```python
from build123d import *

# Parameters (mm, degrees)
ESQUISSE1_W                                       = 60
ESQUISSE1_H                                       = 22.8
BOSS_EXTRU_1_DEPTH                                = 1.5
ESQUISSE2_W                                       = 60
ESQUISSE2_H                                       = 5
BOSS_EXTRU_2_DEPTH                                = 10
ESQUISSE7_W                                       = 60
ESQUISSE7_H                                       = 22.4
BOSS_EXTRU_3_DEPTH                                = 5
DIAM_TRE_DU_PER_AGE_3_0_3_2_AT_2_COUNT            = 2
DIAM_TRE_DU_PER_AGE_3_0_3_2_AT_2_PITCH            = 10
DIAM_TRE_DU_PER_AGE_3_0_3_2_AT_3_COUNT            = 2
DIAM_TRE_DU_PER_AGE_3_0_3_2_AT_3_PITCH            = 20
DIAM_TRE_DU_PER_AGE_3_0_3_2_AT_4_COUNT            = 2
DIAM_TRE_DU_PER_AGE_3_0_3_2_AT_4_PITCH            = 30
DIAM_TRE_DU_PER_AGE_3_0_3_2_AT_5_COUNT            = 2
DIAM_TRE_DU_PER_AGE_3_0_3_2_AT_5_PITCH            = 40
R_P_TITION_LIN_AIRE2_COUNT                        = 2
R_P_TITION_LIN_AIRE2_PITCH                        = 10
CHAMBRAGE_POUR_VIS_SIX_PANS_CREUX_M31_D           = 3.4
CHAMBRAGE_POUR_VIS_SIX_PANS_CREUX_M31_DEPTH       = 13
CHAMBRAGE_POUR_VIS_SIX_PANS_CREUX_M31_CBORE_D     = 6.5
CHAMBRAGE_POUR_VIS_SIX_PANS_CREUX_M31_CBORE_DEPTH = 1
CHAMBRAGE_POUR_VIS_SIX_PANS_CREUX_M31_TIP         = 1.021463052
R_P_TITION_LIN_AIRE1_COUNT                        = 3
R_P_TITION_LIN_AIRE1_PITCH                        = 10
ESQUISSE10_W                                      = 40
ESQUISSE10_H                                      = 32.8
BOSS_EXTRU_4_DEPTH                                = 2
ESQUISSE11_W                                      = 20
ESQUISSE11_H                                      = 10
ENL_V_MAT_EXTRU_1_DEPTH                           = 17.4
ENL_V_MAT_EXTRU_1_DEPTH_BACK                      = 17.4
ESQUISSE12_R                                      = 4
ESQUISSE12_W                                      = 11.5
ESQUISSE12_H                                      = 8
ENL_V_MAT_EXTRU_2_DEPTH                           = 23.9
ENL_V_MAT_EXTRU_2_DEPTH_BACK                      = 12.5
BOSS_EXTRU_5_DEPTH                                = 4
ESQUISSE14_W                                      = 2
ESQUISSE14_H                                      = 8
ENL_V_MAT_EXTRU_3_DEPTH                           = 1
ENL_V_MAT_EXTRU_3_DEPTH_BACK                      = 65
CONG_2_R                                          = 2
ESQUISSE15_W                                      = 14.8
ESQUISSE15_H                                      = 1.5
ENL_V_MAT_EXTRU_4_DEPTH                           = 5
ENL_V_MAT_EXTRU_4_DEPTH_BACK                      = 25
CONG_3_R                                          = 0.5


with BuildPart() as part:
    # Esquisse1 → Boss.-Extru.1 (new body, symmetric)
    with BuildSketch(Plane(origin=(0, 0, 0), x_dir=(1, 0, 0), z_dir=(0, 1, 0))):
        Rectangle(ESQUISSE1_W, ESQUISSE1_H)
    extrude(amount=BOSS_EXTRU_1_DEPTH, both=True)

    # Esquisse2 → Boss.-Extru.2 (add)
    with BuildSketch(Plane.XZ.offset(1.5)):
        Rectangle(ESQUISSE2_W, ESQUISSE2_H)
    extrude(amount=BOSS_EXTRU_2_DEPTH)

    # Esquisse7 → Boss.-Extru.3 (add)
    with BuildSketch(Plane(origin=(0, 0, -11.4), x_dir=(-1, 0, 0), z_dir=(0, 0, -1))):
        with Locations((0, 9.7)):
            Rectangle(ESQUISSE7_W, ESQUISSE7_H)
    boss_extru_3 = extrude(amount=BOSS_EXTRU_3_DEPTH)

    # Esquisse9 → Diamètre du perçage Ø3.0 (3)2 (revolve, cut)
    with BuildSketch(Plane(origin=(20, 4.5, -16.4), x_dir=(0, 1, 0), z_dir=(1, 0, 0))):
        Polygon((0, 0), (0, 13.901290929), (1.5, 13), (1.5, 0), align=None)
    diam_tre_du_per_age_3_0_3_2 = revolve(axis=Axis((20, 4.5, -22.75), (0, 0, 1)), mode=Mode.SUBTRACT)

    # Diamètre du perçage Ø3.0 (3)2 at 2: Diamètre du perçage Ø3.0 (3)2 ×2
    with Locations(*[(-i * DIAM_TRE_DU_PER_AGE_3_0_3_2_AT_2_PITCH, 0, 0) for i in range(1, DIAM_TRE_DU_PER_AGE_3_0_3_2_AT_2_COUNT)]):
        add(diam_tre_du_per_age_3_0_3_2, mode=Mode.SUBTRACT)

    # Diamètre du perçage Ø3.0 (3)2 at 3: Diamètre du perçage Ø3.0 (3)2 ×2
    with Locations(*[(-i * DIAM_TRE_DU_PER_AGE_3_0_3_2_AT_3_PITCH, 0, 0) for i in range(1, DIAM_TRE_DU_PER_AGE_3_0_3_2_AT_3_COUNT)]):
        add(diam_tre_du_per_age_3_0_3_2, mode=Mode.SUBTRACT)

    # Diamètre du perçage Ø3.0 (3)2 at 4: Diamètre du perçage Ø3.0 (3)2 ×2
    with Locations(*[(-i * DIAM_TRE_DU_PER_AGE_3_0_3_2_AT_4_PITCH, 0, 0) for i in range(1, DIAM_TRE_DU_PER_AGE_3_0_3_2_AT_4_COUNT)]):
        add(diam_tre_du_per_age_3_0_3_2, mode=Mode.SUBTRACT)

    # Diamètre du perçage Ø3.0 (3)2 at 5: Diamètre du perçage Ø3.0 (3)2 ×2
    with Locations(*[(-i * DIAM_TRE_DU_PER_AGE_3_0_3_2_AT_5_PITCH, 0, 0) for i in range(1, DIAM_TRE_DU_PER_AGE_3_0_3_2_AT_5_COUNT)]):
        add(diam_tre_du_per_age_3_0_3_2, mode=Mode.SUBTRACT)

    # Répétition linéaire2: Diamètre du perçage Ø3.0 (3)2 ×2
    with Locations(*[(0, i * R_P_TITION_LIN_AIRE2_PITCH, 0) for i in range(1, R_P_TITION_LIN_AIRE2_COUNT)]):
        add(diam_tre_du_per_age_3_0_3_2, mode=Mode.SUBTRACT)

    # Répétition linéaire2 copy 1 sketch → Répétition linéaire2 copy 1 (revolve, cut)
    with BuildSketch(Plane(origin=(10, 14.5, -16.4), x_dir=(0, 1, 0), z_dir=(1, 0, 0))):
        Polygon((0, 0), (0, 13.901290929), (1.5, 13), (1.5, 0), align=None)
    revolve(axis=Axis((10, 14.5, -22.75), (0, 0, 1)), mode=Mode.SUBTRACT)

    # Répétition linéaire2 copy 2 sketch → Répétition linéaire2 copy 2 (revolve, cut)
    with BuildSketch(Plane(origin=(0, 14.5, -16.4), x_dir=(0, 1, 0), z_dir=(1, 0, 0))):
        Polygon((0, 0), (0, 13.901290929), (1.5, 13), (1.5, 0), align=None)
    revolve(axis=Axis((0, 14.5, -22.75), (0, 0, 1)), mode=Mode.SUBTRACT)

    # Répétition linéaire2 copy 3 sketch → Répétition linéaire2 copy 3 (revolve, cut)
    with BuildSketch(Plane(origin=(-10, 14.5, -16.4), x_dir=(0, 1, 0), z_dir=(1, 0, 0))):
        Polygon((0, 0), (0, 13.901290929), (1.5, 13), (1.5, 0), align=None)
    revolve(axis=Axis((-10, 14.5, -22.75), (0, 0, 1)), mode=Mode.SUBTRACT)

    # Répétition linéaire2 copy 4 sketch → Répétition linéaire2 copy 4 (revolve, cut)
    with BuildSketch(Plane(origin=(-20, 14.5, -16.4), x_dir=(0, 1, 0), z_dir=(1, 0, 0))):
        Polygon((0, 0), (0, 13.901290929), (1.5, 13), (1.5, 0), align=None)
    revolve(axis=Axis((-20, 14.5, -22.75), (0, 0, 1)), mode=Mode.SUBTRACT)

    # Symétrie1: Boss.-Extru.3, Diamètre du perçage Ø3.0 (3)2 across plane
    add(boss_extru_3.mirror(Plane.XY))
    add(diam_tre_du_per_age_3_0_3_2.mirror(Plane.XY), mode=Mode.SUBTRACT)

    # Symétrie1 copy 1 sketch → Symétrie1 copy 1 (revolve, cut)
    with BuildSketch(Plane(origin=(20, 14.5, 16.4), x_dir=(0, 1, 0), z_dir=(1, 0, 0))):
        Polygon((0, 0), (0, -13.901290929), (1.5, -13), (1.5, 0), align=None)
    revolve(axis=Axis((20, 14.5, 22.75), (0, 0, 1)), mode=Mode.SUBTRACT)

    # Symétrie1 copy 2 sketch → Symétrie1 copy 2 (revolve, cut)
    with BuildSketch(Plane(origin=(10, 14.5, 16.4), x_dir=(0, 1, 0), z_dir=(1, 0, 0))):
        Polygon((0, 0), (0, -13.901290929), (1.5, -13), (1.5, 0), align=None)
    revolve(axis=Axis((10, 14.5, 22.75), (0, 0, 1)), mode=Mode.SUBTRACT)

    # Symétrie1 copy 3 sketch → Symétrie1 copy 3 (revolve, cut)
    with BuildSketch(Plane(origin=(0, 14.5, 16.4), x_dir=(0, 1, 0), z_dir=(1, 0, 0))):
        Polygon((0, 0), (0, -13.901290929), (1.5, -13), (1.5, 0), align=None)
    revolve(axis=Axis((0, 14.5, 22.75), (0, 0, 1)), mode=Mode.SUBTRACT)

    # Symétrie1 copy 4 sketch → Symétrie1 copy 4 (revolve, cut)
    with BuildSketch(Plane(origin=(-10, 14.5, 16.4), x_dir=(0, 1, 0), z_dir=(1, 0, 0))):
        Polygon((0, 0), (0, -13.901290929), (1.5, -13), (1.5, 0), align=None)
    revolve(axis=Axis((-10, 14.5, 22.75), (0, 0, 1)), mode=Mode.SUBTRACT)

    # Symétrie1 copy 5 sketch → Symétrie1 copy 5 (revolve, cut)
    with BuildSketch(Plane(origin=(-20, 14.5, 16.4), x_dir=(0, 1, 0), z_dir=(1, 0, 0))):
        Polygon((0, 0), (0, -13.901290929), (1.5, -13), (1.5, 0), align=None)
    revolve(axis=Axis((-20, 14.5, 22.75), (0, 0, 1)), mode=Mode.SUBTRACT)

    # Symétrie1 copy 6 sketch → Symétrie1 copy 6 (revolve, cut)
    with BuildSketch(Plane(origin=(10, 4.5, 16.4), x_dir=(0, 1, 0), z_dir=(1, 0, 0))):
        Polygon((0, 0), (0, -13.901290929), (1.5, -13), (1.5, 0), align=None)
    revolve(axis=Axis((10, 4.5, 22.75), (0, 0, 1)), mode=Mode.SUBTRACT)

    # Symétrie1 copy 7 sketch → Symétrie1 copy 7 (revolve, cut)
    with BuildSketch(Plane(origin=(0, 4.5, 16.4), x_dir=(0, 1, 0), z_dir=(1, 0, 0))):
        Polygon((0, 0), (0, -13.901290929), (1.5, -13), (1.5, 0), align=None)
    revolve(axis=Axis((0, 4.5, 22.75), (0, 0, 1)), mode=Mode.SUBTRACT)

    # Symétrie1 copy 8 sketch → Symétrie1 copy 8 (revolve, cut)
    with BuildSketch(Plane(origin=(-10, 4.5, 16.4), x_dir=(0, 1, 0), z_dir=(1, 0, 0))):
        Polygon((0, 0), (0, -13.901290929), (1.5, -13), (1.5, 0), align=None)
    revolve(axis=Axis((-10, 4.5, 22.75), (0, 0, 1)), mode=Mode.SUBTRACT)

    # Symétrie1 copy 9 sketch → Symétrie1 copy 9 (revolve, cut)
    with BuildSketch(Plane(origin=(-20, 4.5, 16.4), x_dir=(0, 1, 0), z_dir=(1, 0, 0))):
        Polygon((0, 0), (0, -13.901290929), (1.5, -13), (1.5, 0), align=None)
    revolve(axis=Axis((-20, 4.5, 22.75), (0, 0, 1)), mode=Mode.SUBTRACT)

    # Esquisse4 → Diamètre du perçage Ø3.0 (3)1 (revolve, cut)
    with BuildSketch(Plane(origin=(-20, -6.5, 2.5), x_dir=(0, -1, 0), z_dir=(1, 0, 0))):
        Polygon((0, 0), (0, 13.901290929), (1.5, 13), (1.5, 0), align=None)
    diam_tre_du_per_age_3_0_3_1 = revolve(axis=Axis((-20, -6.5, 8.85), (0, 0, -1)), mode=Mode.SUBTRACT)

    # Chambrage pour vis à six pans creux M31
    with Locations(Plane(origin=(0, -1.5, 0), x_dir=(-1, 0, 0), z_dir=(0, -1, 0))):
        with Locations((-4, 8.5), (-4, -8.5)):
            CounterBoreHole(CHAMBRAGE_POUR_VIS_SIX_PANS_CREUX_M31_D / 2, CHAMBRAGE_POUR_VIS_SIX_PANS_CREUX_M31_CBORE_D / 2, CHAMBRAGE_POUR_VIS_SIX_PANS_CREUX_M31_CBORE_DEPTH, depth=CHAMBRAGE_POUR_VIS_SIX_PANS_CREUX_M31_DEPTH)
            with Locations((0, 0, -(CHAMBRAGE_POUR_VIS_SIX_PANS_CREUX_M31_DEPTH + CHAMBRAGE_POUR_VIS_SIX_PANS_CREUX_M31_TIP / 2))):  # 118° drill point
                Cone(0, CHAMBRAGE_POUR_VIS_SIX_PANS_CREUX_M31_D / 2, CHAMBRAGE_POUR_VIS_SIX_PANS_CREUX_M31_TIP, mode=Mode.SUBTRACT)

    # Répétition linéaire1: Diamètre du perçage Ø3.0 (3)1 ×3
    with Locations(*[(i * R_P_TITION_LIN_AIRE1_PITCH, 0, 0) for i in range(1, R_P_TITION_LIN_AIRE1_COUNT)]):
        add(diam_tre_du_per_age_3_0_3_1, mode=Mode.SUBTRACT)

    # Esquisse10 → Boss.-Extru.4 (add)
    with BuildSketch(Plane(origin=(0, 20.9, 0), x_dir=(1, 0, 0), z_dir=(0, 1, 0))):
        with Locations((-10, 0)):
            Rectangle(ESQUISSE10_W, ESQUISSE10_H)
    extrude(amount=BOSS_EXTRU_4_DEPTH)

    # Esquisse11 → Enlèv. mat.-Extru.1 (cut, two sides)
    with BuildSketch(Plane.XY) as enl_v_mat_extru_1_sk:
        with Locations((20, -6.5)):
            Rectangle(ESQUISSE11_W, ESQUISSE11_H)
    extrude(amount=ENL_V_MAT_EXTRU_1_DEPTH, mode=Mode.SUBTRACT)
    extrude(enl_v_mat_extru_1_sk.sketch, amount=-ENL_V_MAT_EXTRU_1_DEPTH_BACK, mode=Mode.SUBTRACT)

    # Esquisse12 → Enlèv. mat.-Extru.2 (cut, two sides)
    with BuildSketch(Plane(origin=(0, 0, 0), x_dir=(1, 0, 0), z_dir=(0, 1, 0))) as enl_v_mat_extru_2_sk:
        with Locations((18.5, 0)):
            Circle(ESQUISSE12_R)
        with Locations((24.25, 0)):
            Rectangle(ESQUISSE12_W, ESQUISSE12_H)
    extrude(amount=ENL_V_MAT_EXTRU_2_DEPTH, mode=Mode.SUBTRACT)
    extrude(enl_v_mat_extru_2_sk.sketch, amount=-ENL_V_MAT_EXTRU_2_DEPTH_BACK, mode=Mode.SUBTRACT)

    # Esquisse13 → Boss.-Extru.5 (add)
    with BuildSketch(Plane.ZY.offset(30)):
        Polygon((16.4, 22.9), (-16.4, 22.9), (-16.4, 8.9), (-11.4, 8.9), (-11.4, 20.9), (11.4, 20.9), (11.4, 8.9), (16.4, 8.9), align=None)
        Polygon((-11.4, 20.9), (-11.4, 8.9), (11.359705281, 8.9), (11.4, 8.9), (11.4, 20.9), align=None)
        Polygon((-11.4, 8.9), (-16.4, 8.9), (-16.4, -1.5), (-2.5, -1.5), (-2.5, -11.5), (2.5, -11.5), (2.5, -1.5), (16.4, -1.5), (16.4, 8.9), (11.4, 8.9), (11.4, 1.5), (-11.4, 1.5), align=None)
    extrude(amount=BOSS_EXTRU_5_DEPTH)

    # Esquisse14 → Enlèv. mat.-Extru.3 (cut, two sides)
    with BuildSketch(Plane.ZY.offset(34)) as enl_v_mat_extru_3_sk:
        with Locations((7, 16.010631071)):
            Rectangle(ESQUISSE14_W, ESQUISSE14_H)
        with Locations((-7, 16.010631071)):
            Rectangle(ESQUISSE14_W, ESQUISSE14_H)
    extrude(amount=ENL_V_MAT_EXTRU_3_DEPTH, mode=Mode.SUBTRACT)
    extrude(enl_v_mat_extru_3_sk.sketch, amount=-ENL_V_MAT_EXTRU_3_DEPTH_BACK, mode=Mode.SUBTRACT)

    # Congé2
    cong_2_edges = [part.edges().sort_by_distance(p)[0] for p in [
        (-12, -1.5, -2.5),
        (-12, 22.9, 16.4),
        (-12, 22.9, -16.4),
        (-12, -1.5, 2.5),
        (10, -1.5, 0),
        (30, 0, -4),
        (30, 0, 4),
        (-2, -1.5, -16.4),
        (-2, -1.5, 16.4),
    ]]
    fillet(cong_2_edges, radius=CONG_2_R)

    # Esquisse15 → Enlèv. mat.-Extru.4 (cut, two sides)
    with BuildSketch(Plane.ZY.offset(30)) as enl_v_mat_extru_4_sk:
        with Locations((0, 0.75)):
            Rectangle(ESQUISSE15_W, ESQUISSE15_H)
    extrude(amount=ENL_V_MAT_EXTRU_4_DEPTH, mode=Mode.SUBTRACT)
    extrude(enl_v_mat_extru_4_sk.sketch, amount=-ENL_V_MAT_EXTRU_4_DEPTH_BACK, mode=Mode.SUBTRACT)

    # Congé3
    cong_3_edges = [part.edges().sort_by_distance(p)[0] for p in [
        (-19.5, 1.5, -7.4),
        (-19.5, 0, -7.4),
        (-5, 0, 0),
        (-19.5, 0, 7.4),
        (-19.5, 1.5, 7.4),
        (-5, 1.5, 0),
    ]]
    fillet(cong_3_edges, radius=CONG_3_R)


solid = part.part
```
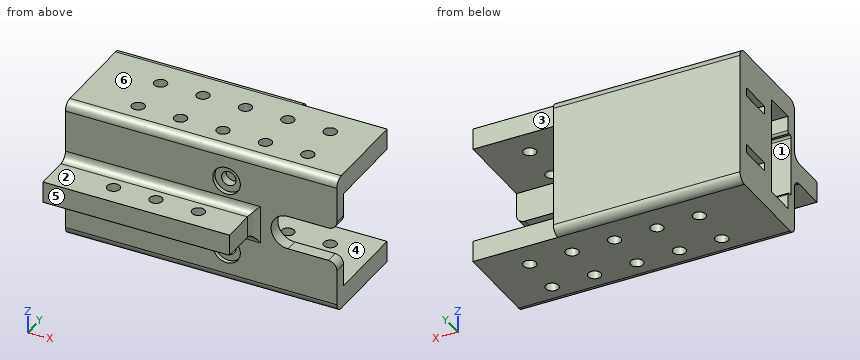
Design review of the part built by this model. Coordinates are the model's own, in mm. Face numbers are marked on the shaded views. A direction names the side the tool comes from. Give positions to 0.01 mm unless a question says otherwise; leave off trailing zeros. Loops run counter-clockwise (first coordinate to the right, second up) from the corner with the lowest first, then second, coordinate; pieces in that order, holes last. Notation, with made-up numbers: M 81.25,32.5 L 116.25,32.5 A15 ccw 116.25,42.5 Z; hole C 69.5,15.5 d2. An arc over 180 degrees is marked long. Return JSON: item names as keys, results as strings. Group by question number.
Item 1: Mouldability with a two-part tool opening along Z and no side actions: class the marked faces 4, 5 and 6 as released by +Z, released by -Z, zero draft, split by the parting line, or undercut.
Item 2: We need section C-C (z = -13). Give the number of separate pieces and of enclosed holes in the cut face, and give its area (3 significant figures).
Item 3: Insertion check: pin 1 Ø2.5 at (x, y) = (0, 4.5) entering from -Z; pin 2 Ø2 at (y, z) = (17, 6.5) entering from +X; pin 3 Ø0.6 at (x, z) = (-32, -6.5) entering from -Y; pin 4 Ø5 at (x, y) = (0, 14.5) entering from -Z. Each pin has a flat end and moves straight along its axis. Give the tip position at first contact, or say it passes through.
Item 4: We need section A-A (y = -6.5). Give the boundary of the cut face in (x, z), and give its area (3 significant figures).
Item 5: For probe 1 along X at (y, z) = (14.5, 14.05); probe 2 along Y at (x, z) = (20, 12.65); probe 3 along X at (y, z) = (-6.5, -0.8), list the stretches that pass through material, from the lowest coordinate up.
Item 6: Tool access review of the marked faces 1, 2 and 3: name each direction out of +Z, -Z, +X, -X, +Y, -Y from which nothing blocks a thin tool from reaching the whole face with its end or side.
Item 7: We need section D-D (x = -7). Give the boundary of the cut face in (y, z), and give its area (3 significant figures).
Output:
{
 "1": {"face 4": "undercut", "face 5": "zero draft", "face 6": "released by +Z"},
 "2": {"separate pieces": "1", "enclosed holes": "10", "area": "1,450 mm^2"},
 "3": {"pin 1": "passes through", "pin 2": "stops at x = -30", "pin 3": "stops at y = -1.5", "pin 4": "stops at z = -16.4"},
 "4": {"outline": "M -34,-2.5 L -21.5,-2.5 L -21.5,2.5 L -34,2.5 Z; M -18.5,-2.5 L -11.5,-2.5 L -11.5,2.5 L -18.5,2.5 Z; M -8.5,-2.5 L -1.5,-2.5 L -1.5,2.5 L -8.5,2.5 Z; M 1.5,-2.5 L 10,-2.5 L 10,2.5 L 1.5,2.5 Z", "area": "175 mm^2"},
 "5": {"probe 1": "x = -34 to -21.5, -18.5 to -11.5, -8.5 to -1.5, 1.5 to 8.5, 11.5 to 18.5, 21.5 to 30", "probe 2": "y = -1.5 to 3, 6 to 13, 16 to 20.9", "probe 3": "x = -34 to -21.5, -18.5 to -11.5, -8.5 to -1.5, 1.5 to 10"},
 "6": {"face 1": "-X", "face 2": "+Z, +X, -X, -Y", "face 3": "+Z, -Z, +X, +Y"},
 "7": {"outline": "M -11.5,-2.5 L -3.5,-2.5 A2 cw -1.5,-4.5 L -1.5,-14.4 A2 ccw 0.5,-16.4 L 20.9,-16.4 A2 ccw 22.9,-14.4 L 22.9,14.4 A2 ccw 20.9,16.4 L 0.5,16.4 A2 ccw -1.5,14.4 L -1.5,4.5 A2 cw -3.5,2.5 L -11.5,2.5 Z; hole M 0,-6.9 A0.5 ccw 0.5,-7.4 L 1,-7.4 A0.5 cw 1.5,-7.9 L 1.5,-11.4 L 20.9,-11.4 L 20.9,11.4 L 1.5,11.4 L 1.5,7.9 A0.5 cw 1,7.4 L 0.5,7.4 A0.5 ccw 0,6.9 Z", "area": "384 mm^2"}
}
